Here's how the part is built. I have some questions about the finished solid (model axes, mm). A direction names the side the tool comes from. Coordinates: 2 decimals unless noted, no trailing zeros. Write each loop counter-clockwise with the first axis right and the second up, starting at its lowest first coordinate (ties: lowest second). Pieces come first, ordered by that corner, then holes. Notation, with made-up numbers: (81, -39.5) -> (98, -39.5) arc R23 cw to (98, -14.5) -> close; hole circle Ø8 at (-38, 27). An arc over 180 degrees is marked (long way). Put each result on its own line as item: value.
```python
from build123d import *

# Parameters (mm, degrees)
F0_R     = 3.81
F1_DEPTH = 2.54
F2_R     = 1.143
F3_DEPTH = 2.54
F5_D     = 1.27
F5_DEPTH = 2.54
F5_TIP   = 0.3815464931
F6_SIZE  = 0.762


with BuildPart() as f1:
    # F0 (on Top) → F1 (new body)
    with BuildSketch(Plane.XY):
        Circle(F0_R)
    extrude(amount=F1_DEPTH)

    # F2 (on face) → F3 (join)
    with BuildSketch(Plane.XY.offset(2.54)):
        Circle(F2_R)
    extrude(amount=F3_DEPTH)

    # F5
    with Locations(Plane(origin=(0, 0, 0), x_dir=(1, 0, 0), z_dir=(0, 0, -1))):
        with Locations((0, 0)):
            Hole(F5_D / 2, depth=F5_DEPTH)
            with Locations((0, 0, -(F5_DEPTH + F5_TIP / 2))):  # 118° drill point
                Cone(0, F5_D / 2, F5_TIP, mode=Mode.SUBTRACT)

    # F6
    f6_edges = [f1.edges().sort_by_distance(p)[0] for p in [
        (-3.81, 0, 0),
    ]]
    chamfer(f6_edges, length=F6_SIZE)


solid = f1.part
```
Item 1: Imagine slicing it at B-B on z = 4.45. Write out the boundary of the cut face in (x, y), then the cut area to 3 significant figures.
Output:
outline: circle Ø2.29 at (0, 0)
area: 4.10 mm²
Item 2: Which directions (+Z, -Z, +X, -X, +Y, -Y) give clear straight access to the entire face, cutting with the end or side of a thin tool? Please do faces 4 (the flat face through (0, 0, 5.08)), 5 (the cylindrical face through (-0.248, -1.116, 3.792)).
Output:
face 4: +Z, +X, -X, +Y, -Y
face 5: +Z
Item 3: Imagine slicing it at A-A on z = 1.3. Write out the boundary of the cut face in (x, y) (3 decimals), then the cut area to 3 significant figures.
Output:
outline: circle Ø7.62 at (0, 0); hole circle Ø1.27 at (0, 0)
area: 44.3 mm²
Item 4: If we mould it in two halves opening along Y, with no side actions, what happens to faces 1 (the cylindrical face through (0.08, -0.63, 1.29)), 2 (the cylindrical face through (-0.83, -3.72, 1.64)), 3 (the flat face through (0, -1, 0))? For each: released by +Y, released by -Y, zero draft, split by the parting line, or undercut.
Output:
face 1: undercut
face 2: split by the parting line
face 3: zero draft
Item 5: For P1, Ø1, axis at x = 0, y = 0, coming from the -Z side; P2, Ø3, axis at x = -2.5, z = 1.5, coming from the +Y side; P3, Ø2, axis at x = -3, y = -1.5, coming from the +Z side, each with a flat end and sliding along its axis, tell me the tip position at first contact or that it passes through.
Output:
P1: stops at z = 2.62
P2: stops at y = 3.68
P3: stops at z = 2.54
Item 6: Please list where these lines run through material, in increasing order: line 1 along Y through (x, z) = (0, 1.4) (3 decimals); line 2 along Z through (x, y) = (-2.5, -1.5); line 3 along X through (y, z) = (0.5, 1.85). Write a range as from..to.
Output:
line 1: y = -3.81..-0.635, 0.635..3.81
line 2: z = 0..2.54
line 3: x = -3.78..-0.39, 0.39..3.78
